Drawing for the job (mm, zero at the part's lowest x, y, z). Round coordinates to 2 decimals unless told otherwise and drop trailing zeros. Loops run counter-clockwise (first coordinate to the right, second up) from the corner with the lowest first, then second, coordinate; pieces in that order, holes last. Notation, with made-up numbers: M 27,21 L 58,21 A25 ccw 58,48 Z; hole C 17,-7.75 d3. An arc over 180 degrees is marked long. Answer in a Markdown table with one row per item.
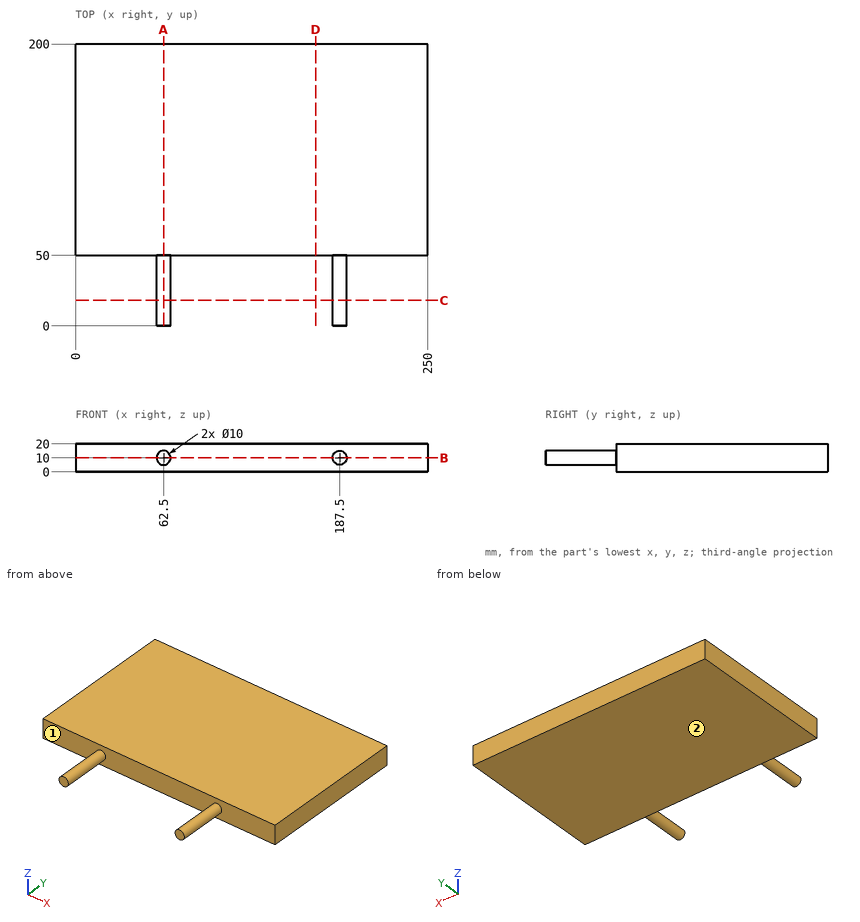
1. Saw through at B-B (z = 10). Write the cut outline in (x, y), and give its area (3 significant figures).
Verdict:
| item | result |
|---|---|
| outline | M 0,50 L 57.5,50 L 57.5,0 L 67.5,0 L 67.5,50 L 182.5,50 L 182.5,0 L 192.5,0 L 192.5,50 L 250,50 L 250,200 L 0,200 Z |
| area | 38,500 mm² |
2. Saw through at A-A (x = 62.5). Write the cut outline in (y, z), and give its area (3 significant figures).
Verdict:
| item | result |
|---|---|
| outline | M 0,5 L 50,5 L 50,0 L 200,0 L 200,20 L 50,20 L 50,15 L 0,15 Z |
| area | 3,500 mm² |
3. Wall check: probe 1 along Y at (x, z) = (236, 13.5); probe 2 along X at (y, z) = (9.5, 8.25). Give the ranges that are in metal, low to high.
Verdict:
| item | result |
|---|---|
| probe 1 | y = 50 to 200 |
| probe 2 | x = 57.82 to 67.18, 182.82 to 192.18 |
4. Mould opens along X. For the marked faces 1 and 2 say: +X half, -X half, draft (parallel to the pull), parting line (faces both ways), or undercut.
Verdict:
| item | result |
|---|---|
| face 1 | undercut |
| face 2 | draft |
5. Pin check, flat tips, straight feed: pin 1 (1.5 mm diameter, centred on x = 204, y = 60, fed in from -Z); pin 2 (1.5 mm diameter, centred on x = 149.5, z = 11, fed in from -Y); pin 3 (3 mm diameter, centred on y = 23, z = 14.5, fed in from -X); pin 4 (4 mm diameter, centred on x = 131.5, y = 47, fed in from +Z). Stop position of each tip, or through.
Verdict:
| item | result |
|---|---|
| pin 1 | stops at z = 0 |
| pin 2 | stops at y = 50 |
| pin 3 | stops at x = 58.5 |
| pin 4 | passes through |
6. Saw through at D-D (x = 170.5). Write the cut outline in (y, z).
Verdict:
| item | result |
|---|---|
| outline | M 50,0 L 200,0 L 200,20 L 50,20 Z |
7. Saw through at C-C (y = 18). Write the cut outline in (x, z).
Verdict:
| item | result |
|---|---|
| outline | C 62.5,10 d10; C 187.5,10 d10 |
